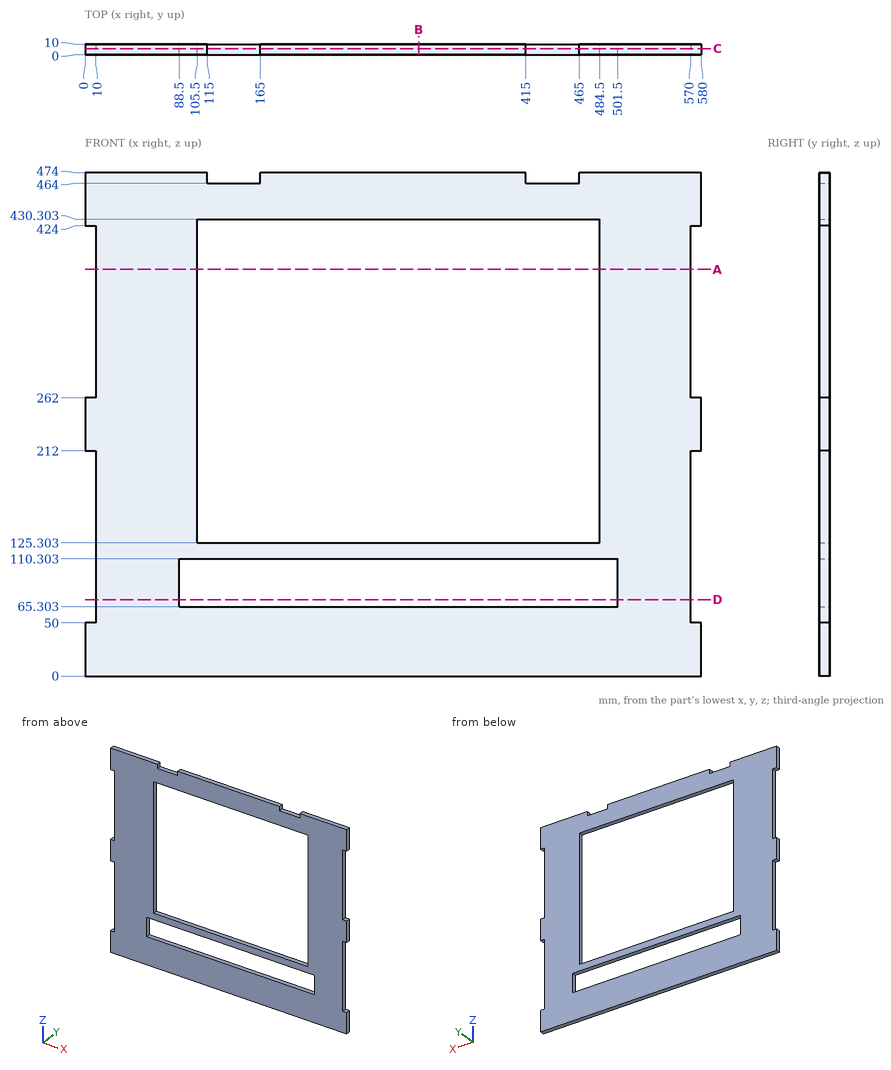
Here's the drawing with two shaded views (mm, measured from the low corner). I have some questions. Give positions to 0.01 mm unless a question says otherwise; leave off trailing zeros. Order: outer loops, then holes, each group sorted by start corner. A loop starts at its lowest first (then second) coordinate and runs counter-clockwise, first axis right, second up.
Q1. Suppose I cut it at C-C, the plane y = 5.75. Count the separate pieces of the cut face and the enclosed holes in it, and give its area (3 significant figures).
Q2. Suppose I cut it at D-D, the plane z = 72. Write out the boundary of the cut face in (x, y).
Q3. Suppose I cut it at B-B, the plane x = 314. Write out the boundary of the cut face in (y, z).
Q4. If I drill on line 1 along Z through (x, y) = (477.5, 4.25); line 2 along Z through (x, y) = (117, 3.25); line 3 along X through (y, z) = (6.25, 93), over which ranges is the centre line in solid material (lowest first)?
Q5. Suppose I cut it at A-A, the plane z = 383. Write out the boundary of the cut face in (x, y), and give its area (3 significant figures).
Q6. I'm going to push flat-ended pins straight in: P1, Ø5, axis at y = 4, z = 308.5, coming from the -X side; P2, Ø5, axis at y = 5.5, z = 94.5, coming from the +X side; P3, Ø3, axis at x = 139.5, y = 3.5, coming from the +Z side. Where does each tip first touch, or does it pass through?
Solution:
1. separate pieces: 1
1. enclosed holes: 2
1. area: 133,000 mm2
2. outline: (10, 0) - (88.5, 0) - (88.5, 10) - (10, 10) - close; (501.5, 0) - (570, 0) - (570, 10) - (501.5, 10) - close
3. outline: (0, 0) - (10, 0) - (10, 65.3) - (0, 65.3) - close; (0, 110.3) - (10, 110.3) - (10, 125.3) - (0, 125.3) - close; (0, 430.3) - (10, 430.3) - (10, 474) - (0, 474) - close
4. line 1: z = 0 to 65.3, 110.3 to 125.3, 430.3 to 474
4. line 2: z = 0 to 65.3, 110.3 to 125.3, 430.3 to 464
4. line 3: x = 10 to 88.5, 501.5 to 570
5. outline: (10, 0) - (105.5, 0) - (105.5, 10) - (10, 10) - close; (484.5, 0) - (570, 0) - (570, 10) - (484.5, 10) - close
5. area: 1,810 mm2
6. P1: stops at x = 10
6. P2: stops at x = 570
6. P3: stops at z = 464
